The model under review builds one solid part; all positions refer to its coordinate system, in mm. A direction names the side the tool comes from. Coordinates: 2 decimals unless noted, no trailing zeros. Write each loop counter-clockwise with the first axis right and the second up, starting at its lowest first coordinate (ties: lowest second). Pieces come first, ordered by that corner, then holes. Notation, with made-up numbers: (-20.75, -22.5) -> (-16.75, -22.5) arc R18 cw to (-16.75, -17.5) -> close; hole circle Ø7 at (35.25, -36). An arc over 180 degrees is marked (long way). Write each question's results on one line, items separated by ' | '.
```python
from build123d import *

# Parameters (mm, degrees)
EXTRUDE1_DEPTH                    = 20
FILLET1_R                         = 2
CHAMFER2_SIZE                     = 1
F_1_4_20_TAPPED_HOLE1_D           = 5.1054
F_1_4_20_TAPPED_HOLE1_DEPTH       = 19.05
F_1_4_20_TAPPED_HOLE1_CSINK_D     = 6.858
F_1_4_20_TAPPED_HOLE1_CSINK_ANGLE = 90
F_1_4_20_TAPPED_HOLE1_TIP         = 1.533816902
CIRPATTERN2_COUNT                 = 4
BOSS_EXTRUDE3_START               = -22
SKETCH11_R                        = 3
BOSS_EXTRUDE3_DEPTH               = 25
CIRPATTERN3_COUNT                 = 4


with BuildPart() as part:
    # Sketch1 → Revolve1 (revolve)
    with BuildSketch(Plane(origin=(0, 0, 0), x_dir=(0, 0, -1), z_dir=(1, 0, 0)), mode=Mode.PRIVATE) as revolve1_sk:
        with BuildLine():
            Line((-96.8, 0), (178.8, 0))
            Line((178.8, 0), (178.8, 4.25))
            Line((178.8, 4.25), (174.1, 4.25))
            Line((174.1, 4.25), (174.1, 6.3))
            Line((174.1, 6.3), (173.1, 6.3))
            Line((173.1, 6.3), (173.1, 40.8))
            Line((173.1, 40.8), (170.1, 40.8))
            Line((170.1, 40.8), (170.1, 37.8))
            Line((170.1, 37.8), (169.6, 37.8))
            Line((169.6, 37.8), (169.6, 40.8))
            Line((169.6, 40.8), (158.2, 40.8))
            Line((158.2, 40.8), (158.2, 37.8))
            Line((158.2, 37.8), (157.7, 37.8))
            Line((157.7, 37.8), (157.7, 40.8))
            Line((157.7, 40.8), (154.7, 40.8))
            Line((154.7, 40.8), (154.7, 6.3))
            Line((154.7, 6.3), (137.7, 6.3))
            Line((137.7, 6.3), (137.7, 7))
            Line((137.7, 7), (135.7, 7))
            Line((135.7, 7), (135.7, 41.5))
            Line((135.7, 41.5), (125.7, 41.5))
            Line((125.7, 41.5), (124.2, 40))
            Line((124.2, 40), (122.7, 41.5))
            Line((122.7, 41.5), (44.7, 41.5))
            Line((44.7, 41.5), (43.7, 40.5))
            Line((43.7, 40.5), (42.7, 41.5))
            Line((42.7, 41.5), (33.7, 41.5))
            Line((33.7, 41.5), (31.7, 39.5))
            Line((31.7, 39.5), (31.7, 34.495478903))
            ThreePointArc((31.7, 34.495478903), (31.432050808, 33.495478903), (30.7, 32.763428096))
            Line((30.7, 32.763428096), (19.2, 26.1239))
            Line((19.2, 26.1239), (1, 26.1239))
            Line((1, 26.1239), (-0.25383158, 25.4))
            Line((-0.25383158, 25.4), (-15.757814772, 25.4))
            Line((-15.757814772, 25.4), (-19, 37.5))
            Line((-19, 37.5), (-22, 37.5))
            Line((-22, 37.5), (-22, 26.15))
            Line((-22, 26.15), (-19.5, 26.15))
            Line((-19.5, 26.15), (-19.5, 23.7109))
            Line((-19.5, 23.7109), (0, 23.7109))
            Line((0, 23.7109), (0, 14))
            Line((0, 14), (-20, 14))
            Line((-20, 14), (-20, 9.525))
            Line((-20, 9.525), (-63, 9.525))
            Line((-63, 9.525), (-63, 12.7))
            Line((-63, 12.7), (-96.8, 12.7))
            Line((-96.8, 12.7), (-96.8, 0))
        make_face()
    revolve(revolve1_sk.sketch.rotate(Axis((0, 0, 96.8), (0, 0, 1)), 90), axis=Axis((0, 0, 96.8), (0, 0, 1)))

    # Sketch2 → Extrude1 (cut, symmetric)
    with BuildSketch(Plane(origin=(0, 0, 0), x_dir=(0, 0, -1), z_dir=(1, 0, 0))):
        Polygon((-81.3, 20), (-81.3, 9.55), (-111.3, 9.55), (-111.3, -9.55), (-81.3, -9.55), (-81.3, -20), (-121.3, -20), (-121.3, 20), align=None)
    extrude(amount=EXTRUDE1_DEPTH, both=True, mode=Mode.SUBTRACT)

    # Fillet1
    fillet1_edges = [part.edges().sort_by_distance(p)[0] for p in [
        (9.525, 0, 20),
        (9.525, 0, 63),
    ]]
    fillet(fillet1_edges, radius=FILLET1_R)

    # Chamfer2
    chamfer2_edges = [part.edges().sort_by_distance(p)[0] for p in [
        (41.5, 0, -135.7),
    ]]
    chamfer(chamfer2_edges, length=CHAMFER2_SIZE)

    # 1_4-20 Tapped Hole1
    with Locations(Plane.XY.offset(96.8)):
        with Locations((-0.077364806, 0.560541021)):
            CounterSinkHole(F_1_4_20_TAPPED_HOLE1_D / 2, F_1_4_20_TAPPED_HOLE1_CSINK_D / 2, depth=F_1_4_20_TAPPED_HOLE1_DEPTH, counter_sink_angle=F_1_4_20_TAPPED_HOLE1_CSINK_ANGLE)
            with Locations((0, 0, -(F_1_4_20_TAPPED_HOLE1_DEPTH + F_1_4_20_TAPPED_HOLE1_TIP / 2))):  # 118° drill point
                Cone(0, F_1_4_20_TAPPED_HOLE1_D / 2, F_1_4_20_TAPPED_HOLE1_TIP, mode=Mode.SUBTRACT)

    # Sketch9 → M4x0.7 Tapped Hole1 (revolve, cut)
    with BuildSketch(Plane(origin=(29.344931419, 29.344931419, -130.7), x_dir=(-0.7071067811865489, 0.7071067811865462, 0), z_dir=(0, 0, 1))):
        Polygon((0, 0), (0, 10.991420021), (1.65, 10), (1.65, 0), align=None)
    m4x0_7_tapped_hole1 = revolve(axis=Axis((33.83505948, 33.83505948, -130.7), (-0.7071067811865462, -0.7071067811865489, 0)), mode=Mode.SUBTRACT)

    # Sketch10 → M4x0.7 Tapped Hole2 (revolve, cut)
    with BuildSketch(Plane(origin=(29.344931419, 29.344931419, -36.7), x_dir=(-0.7071067811865488, 0.7071067811865462, 0), z_dir=(0, 0, 1))):
        Polygon((0, 0), (0, 11.091420021), (1.65, 10.1), (1.65, 0), align=None)
    m4x0_7_tapped_hole2 = revolve(axis=Axis((33.83505948, 33.83505948, -36.7), (-0.7071067811865464, -0.7071067811865488, 0)), mode=Mode.SUBTRACT)

    # CirPattern2: M4x0.7 Tapped Hole1, M4x0.7 Tapped Hole2 ×4 about axis
    cirpattern2_axis = Axis((0, 0, -80.9), (0, 0, 1))
    add([m4x0_7_tapped_hole1.rotate(cirpattern2_axis, i * 360 / CIRPATTERN2_COUNT) for i in range(1, CIRPATTERN2_COUNT)], mode=Mode.SUBTRACT)
    add([m4x0_7_tapped_hole2.rotate(cirpattern2_axis, i * 360 / CIRPATTERN2_COUNT) for i in range(1, CIRPATTERN2_COUNT)], mode=Mode.SUBTRACT)

    # Sketch11 → Boss-Extrude3 (add)
    with BuildSketch(Plane(origin=(0, 0, -173.1), x_dir=(-1, 0, 0), z_dir=(0, 0, -1)).offset(BOSS_EXTRUDE3_START)):
        with Locations((-17.9959, 31.169813128)):
            Circle(SKETCH11_R)
    boss_extrude3 = extrude(amount=BOSS_EXTRUDE3_DEPTH)

    # CirPattern3: Boss-Extrude3 ×4 about axis
    cirpattern3_axis = Axis((0, 0, 0), (0, 0, 1))
    for i in range(1, CIRPATTERN3_COUNT):
        add(boss_extrude3.rotate(cirpattern3_axis, i * 360 / CIRPATTERN3_COUNT))


solid = part.part
```
Q1. Add section A-A (z = 66.5). Write out the cut boundary in (x, y).
Solution:
outline: circle Ø25.4 at (0, 0)
Q2. Clearance check with flat-ended pins moving along their axes: P1, Ø3, axis at x = -32.5, y = 21.5, coming from the -Z side; P2, Ø3.5, axis at x = 0, y = -11.5, coming from the +Z side; P3, Ø2, axis at x = -17.5, y = 26.5, coming from the +Z side. State where each tip first meets the part, or that it passes through.
Solution:
P1: z = -176.1 | P2: z = 81.3 | P3: z = 22
Q3. Machinability: for faces 4 (the cylindrical face through (0.255, 3.092, 86.71)), 5 (the flat face through (-8, -1, -154.7)), 6 (the cylindrical face through (-9.41, 36.61, -157.95)), which of the approach directions +Z, -Z, +X, -X, +Y, -Y give a long, thin tool a straight path to every point of the face, cutting with its end or side? Answer none if there is none.
Solution:
face 4: +Z | face 5: none | face 6: +Y
Q4. Add section B-B (z = -64). Write out the cut boundary in (x, y), plus the area to 3 significant figures.
Solution:
outline: circle Ø83 at (0, 0) | area: 5,410 mm²
Q5. Draft analysis for pull direction Z (two halves, no side actions). For faces 1 (the flat face through (26, 8, 22)), 2 (the cylindrical face through (-25.61, 26.11, -129.09)), 3 (the cylindrical face through (0.553, -4.214, -176.417)), state which applies: pulls with the +Z half, pulls with the -Z half, needs draft (parallel to the pull), parting line crosses it, or undercut.
Solution:
face 1: pulls with the +Z half | face 2: undercut | face 3: needs draft
Q6. For line 1 (Z direction, x = -36.5, y = -10); line 2 (Z direction, x = 13, y = 9); line 3 (Z direction, x = -24.5, y = -20.5), list the stretches that pass through material, from the lowest coordinate up. Write a range as from..to.
Solution:
line 1: -173.1..-170.1, -169.6..-158.2, -157.7..-154.7, -135.7..-31.7 | line 2: -173.1..-154.7, -135.7..0 | line 3: -173.1..-154.7, -135.7..-29.28, 17.51..22
